```python
from build123d import *

# Parameters (mm, degrees)
F0_W     = 31.8
F0_H     = 15.8
F1_DEPTH = 2.5
F2_R     = 2.4
F3_DEPTH = 1.7


with BuildPart() as f1:
    # F0 (on Top) → F1 (new body)
    with BuildSketch(Plane.XY):
        Rectangle(F0_W, F0_H)
    extrude(amount=F1_DEPTH)

    # F2 (on face) → F3 (join)
    with BuildSketch(Plane.XY.offset(2.5)):
        with Locations((-12, 4)):
            Circle(F2_R)
        with Locations((-12, -3.8)):
            Circle(F2_R)
        with Locations((-4.1, -3.8)):
            Circle(F2_R)
        with Locations((-4.1, 4)):
            Circle(F2_R)
        with Locations((3.8, 4)):
            Circle(F2_R)
        with Locations((11.7, -3.8)):
            Circle(F2_R)
        with Locations((11.7, 4)):
            Circle(F2_R)
        with Locations((3.8, -3.8)):
            Circle(F2_R)
    extrude(amount=F3_DEPTH)


solid = f1.part
```
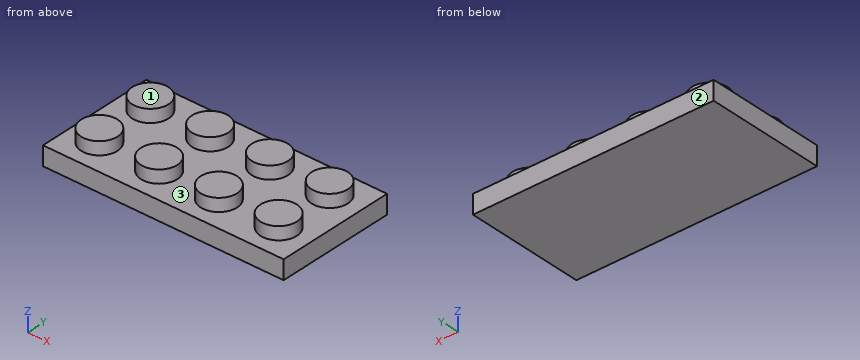
Check sheet for the modelled part. Datum: model origin and axes. Units: mm. Face numbers are marked on the shaded views. Coordinates: 2 decimals unless noted, no trailing zeros. Loops run counter-clockwise (first coordinate to the right, second up) from the corner with the lowest first, then second, coordinate; pieces in that order, holes last. Notation, with made-up numbers: M -27.75,-37 L -20.75,-37 A24 ccw -20.75,-18 Z; hole C 35,21.25 d1. An arc over 180 degrees is marked long. Answer as a JSON object with one key per item and string values.
1. Sectioned sample at A-A on z = 3.45. Record the cut outline in (x, y), and give its area (3 significant figures).
Outcome:
{"outline": "C -12,-3.8 d4.8; C -12,4 d4.8; C -4.1,-3.8 d4.8; C -4.1,4 d4.8; C 3.8,-3.8 d4.8; C 3.8,4 d4.8; C 11.7,-3.8 d4.8; C 11.7,4 d4.8", "area": "145 mm²"}
2. Release check for a two-part mould opening along Y. For the marked faces 1, 2 and 3 record: pulls with the +Y half, pulls with the -Y half, needs draft (parallel to the pull), parting line crosses it, or undercut.
Outcome:
{"face 1": "needs draft", "face 2": "pulls with the +Y half", "face 3": "undercut"}
3. Sectioned sample at C-C on y = -3.8. Record the cut outline in (x, z).
Outcome:
{"outline": "M -15.9,0 L 15.9,0 L 15.9,2.5 L 14.1,2.5 L 14.1,4.2 L 9.3,4.2 L 9.3,2.5 L 6.2,2.5 L 6.2,4.2 L 1.4,4.2 L 1.4,2.5 L -1.7,2.5 L -1.7,4.2 L -6.5,4.2 L -6.5,2.5 L -9.6,2.5 L -9.6,4.2 L -14.4,4.2 L -14.4,2.5 L -15.9,2.5 Z"}
4. Sectioned sample at D-D on x = -14. Record the cut outline in (y, z).
Outcome:
{"outline": "M -7.9,0 L 7.9,0 L 7.9,2.5 L 5.33,2.5 L 5.33,4.2 L 2.67,4.2 L 2.67,2.5 L -2.47,2.5 L -2.47,4.2 L -5.13,4.2 L -5.13,2.5 L -7.9,2.5 Z"}
5. Scan lines: L1, parallel to X at y = -3, z = 3.35; L2, parallel to X at y = 2.25, z = 3.3; L3, parallel to Z at x = -1.5, y = -4. Record each from-to range of solid material in increasing order. Write a range as from..to.
Outcome:
{"L1": "-14.26..-9.74, -6.36..-1.84, 1.54..6.06, 9.44..13.96", "L2": "-13.64..-10.36, -5.74..-2.46, 2.16..5.44, 10.06..13.34", "L3": "0..2.5"}
6. Sectioned sample at B-B on x = 3.8. Record the cut outline in (y, z).
Outcome:
{"outline": "M -7.9,0 L 7.9,0 L 7.9,2.5 L 6.4,2.5 L 6.4,4.2 L 1.6,4.2 L 1.6,2.5 L -1.4,2.5 L -1.4,4.2 L -6.2,4.2 L -6.2,2.5 L -7.9,2.5 Z"}
